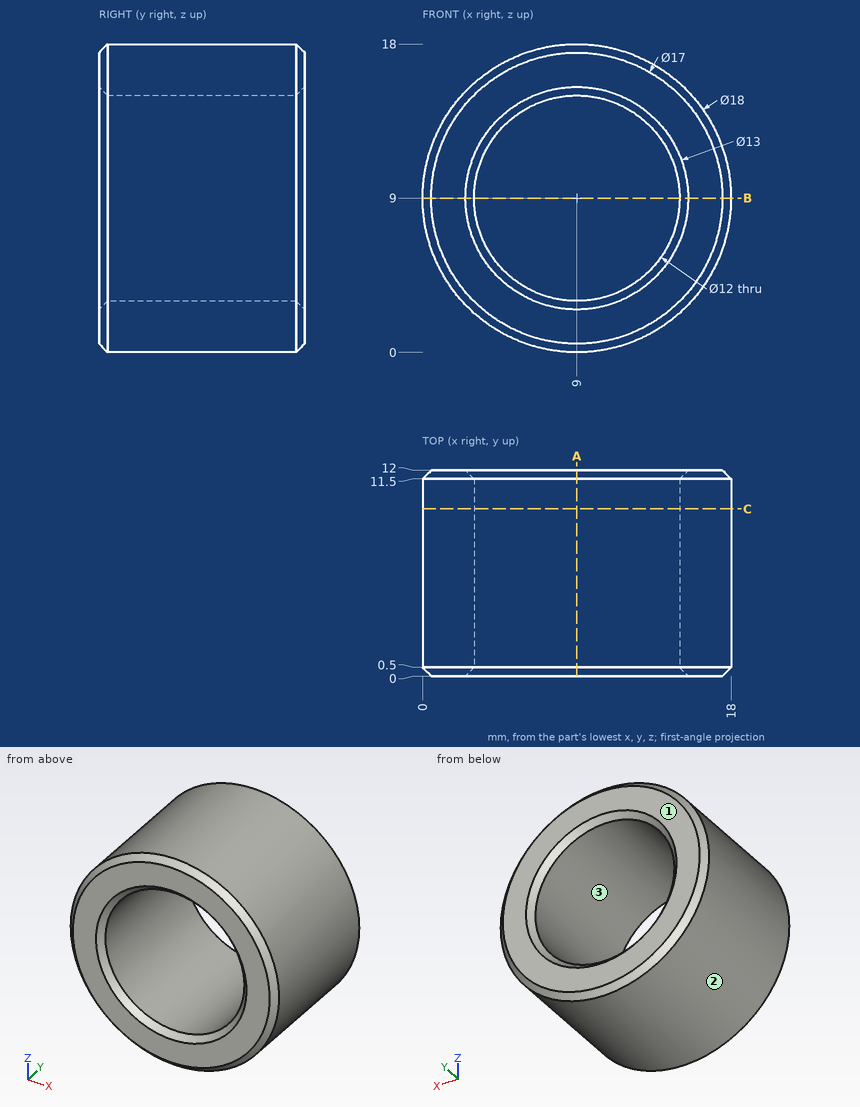
Study the drawing (mm; zero at the part's minimum x, y, z) and answer. Round coordinates to 2 decimals unless told otherwise and drop trailing zeros. Write each loop counter-clockwise with the first axis right and the second up, starting at its lowest first coordinate (ties: lowest second). Pieces come first, ordered by that corner, then holes. Notation, with made-up numbers: (88.5, -35.75) - (109.5, -35.75) arc R11 cw to (109.5, -14.75) - close; hole circle Ø11 at (-24.5, -11). An arc over 180 degrees is marked (long way). Use a Markdown table: item, result. Add a question column.
1. Consider line 1 (X direction, y = 6.5, z = 9); line 2 (Z direction, x = 4, y = 7.5); line 3 (X direction, y = 2.75, z = 10.25). Determine where each line is inside the solid, lowest interval first.
2. The part is cut by section B-B (z = 9). Write down the section's boundary in (x, y).
3. Flat-ended cylindrical pins translate along their axes: P1, Ø1, axis at x = 16, y = 6, coming from the +Z side; P2, Ø3, axis at x = 13.5, y = 9, coming from the +Z side; P3, Ø1.5, axis at x = 12, y = 2.5, coming from the -Z side. Find the tip coordinate at first contact, or state that the pin passes through.
4. The part is cut by section A-A (x = 9). Write down the section's boundary in (y, z).
5. For a pull along Z with two mould halves and no side action, classify the marked faces 1, 2 and 3 as +Z half, -Z half, draft (parallel to the pull), parting line (faces both ways), or undercut.
6. The part is cut by section C-C (y = 9.75). Write down the section's boundary in (x, z), and give its area (3 significant figures).
Reported:
| question | item | result |
|---|---|---|
| 1 | line 1 | 0 to 3, 15 to 18 |
| 1 | line 2 | 1.52 to 5.68, 12.32 to 16.48 |
| 1 | line 3 | 0.09 to 3.13, 14.87 to 17.91 |
| 2 | outline | (0, 0.5) - (0.5, 0) - (2.5, 0) - (3, 0.5) - (3, 11.5) - (2.5, 12) - (0.5, 12) - (0, 11.5) - close; (15, 0.5) - (15.5, 0) - (17.5, 0) - (18, 0.5) - (18, 11.5) - (17.5, 12) - (15.5, 12) - (15, 11.5) - close |
| 3 | P1 | z = 15.22 |
| 3 | P2 | z = 17.49 |
| 3 | P3 | z = 0.29 |
| 4 | outline | (0, 0.5) - (0.5, 0) - (11.5, 0) - (12, 0.5) - (12, 2.5) - (11.5, 3) - (0.5, 3) - (0, 2.5) - close; (0, 15.5) - (0.5, 15) - (11.5, 15) - (12, 15.5) - (12, 17.5) - (11.5, 18) - (0.5, 18) - (0, 17.5) - close |
| 5 | face 1 | draft |
| 5 | face 2 | parting line |
| 5 | face 3 | undercut |
| 6 | outline | circle Ø18 at (9, 9); hole circle Ø12 at (9, 9) |
| 6 | area | 141 mm^2 |
